Geometry: final body of the model. Coordinates: model frame, mm. A direction names the side the tool comes from. Coordinates: 2 decimals unless noted, no trailing zeros. Order: outer loops, then holes, each group sorted by start corner. A loop starts at its lowest first (then second) coordinate and runs counter-clockwise, first axis right, second up. Notation, with made-up numbers: (73, -4) -> (111, -4) arc R13 ccw to (111, 10) -> close; hole circle Ø5 at (41, 15.25). An arc over 180 degrees is marked (long way). Answer in a Markdown table with one row per item. Add a question column.
1) Set-up query: faces 5 (the face through (-2.41, 1.52, 11.2)), 6 (the face through (-0.066, -3.15, 6.785)), 7 (the face through (0, 2.2, 6.5)). Return all of +Z, -Z, +X, -X, +Y, -Y with unobstructed straight access to the full face (end or side cutting, diameter ignored); none if empty.
2) Section query B-B on z = 2.75. Return the cut outline in (x, y), then the cut area to 3 significant figures.
3) Contact query for flat-ended pins moving along their axis: P1, Ø1.5, axis at x = -3, z = 6.5, coming from the -Y side; P2, Ø1, axis at y = -3.5, z = 2, coming from the -X side; P3, Ø4, axis at x = -3, z = 12.5, coming from the -Y side. Output: stop coordinate, or through.
4) Pull-direction query (X, two-part tool) for faces 1 (the face through (-2.761, -1.518, 6.785)), 2 (the face through (1.95, 0, 3)), 3 (the face through (0, 2.8, 3.2)), 4 (the face through (-3, 3, 6.5)); classes: +X half, -X half, draft (parallel to the pull), parting line (faces both ways), or undercut.
5) Section query A-A on z = 10.25. Return the cut outline in (x, y).
6) Ray query, line 1 (X direction, y = 0, z = 10.5); line 2 (Y direction, x = 0, z = 12); line 3 (Z direction, x = 1.75, y = -4). Return the intervals inside material, ascending. Write a range as from..to.
Autodesk Fusion 360 part; units mm, degrees
sketch "Skizze1" plane through (0, 0, 0) normal (0, 0, 1) x (1, 0, 0)
  circle A0 centre (0, 0) radius 2.8
  circle A1 centre (0, 0) radius 5
  line L0 (1.95, -2.0094) -> (-1.95, -2.0094)
  line L1 (-1.95, -2.0094) -> (-1.95, 2.0094)
  line L2 (-1.95, 2.0094) -> (1.95, 2.0094)
  line L3 (1.95, 2.0094) -> (1.95, -2.0094)
  line L4 (1.95, -2.0094) -> (-1.95, 2.0094) construction
  line L5 (-1.95, -2.0094) -> (1.95, 2.0094) construction
  dimension "d1" = 5.6
  dimension "d2" = 10
  dimension "d3" = 3.9
extrude "Extrusion1" add sketch "Skizze1" along normal blind 6.5 contours A0 L3 | A0 L1 | A1 makes body 1
ref_plane "Arbeitsebene1" through (0, 0, 6.5) normal (0, 0, 1) x (1, 0, 0)
sketch "Skizze2" plane through (0, 0, 6.5) normal (0, 0, 1) x (1, 0, 0)
  line L0 (-3.2893, 0.101) -> (-1.7322, -2.7981)
  line L1 (-1.7322, -2.7981) -> (1.5572, -2.8992)
  line L2 (1.5572, -2.8992) -> (3.2893, -0.101)
  line L3 (3.2893, -0.101) -> (1.7322, 2.7981)
  line L4 (1.7322, 2.7981) -> (-1.5572, 2.8992)
  line L5 (-1.5572, 2.8992) -> (-3.2893, 0.101)
  dimension "d7" = 2.85
extrude "Extrusion2" add sketch "Skizze2" along normal blind 10.5 separate body makes body 2
sketch "Skizze3" plane through (0, 0, 17) normal (0, 0, 1) x (-1, 0, 0)
  line L0 (1.5572, -2.8992) -> (3.2893, -0.101)
  line L1 (3.2893, -0.101) -> (1.7322, 2.7981)
  line L2 (1.7322, 2.7981) -> (-1.5572, 2.8992)
  line L3 (-1.5572, 2.8992) -> (-3.2893, 0.101)
  line L4 (-3.2893, 0.101) -> (-1.7322, -2.7981)
  line L5 (-1.7322, -2.7981) -> (1.5572, -2.8992)
  circle A0 centre (0, 0) radius 2
  dimension "d10" = 4
extrude "Extrusion3" cut sketch "Skizze3" against normal blind 10.5 contours A0 bodies 2
combine "Kombinieren1" operation add target body 1 tool bodies 2
fillet "Abrundung1" radius 1 6 edges at (2.4233, -1.5001, 6.5) (2.5108, 1.3485, 6.5) (0.0875, 2.8487, 6.5) (-0.0875, -2.8487, 6.5) (-2.5108, -1.3485, 6.5) (-2.4233, 1.5001, 6.5) on bodies 1
extrude "Extrusion4" cut 1 faces at (-0.1082, -2.5639, 17) along direction (0, 0, -1) blind 2 on bodies 1 bodies 1
equation "d7 = ( 5.7 / 2 ) * 1 mm"
Result:
| question | item | result |
|---|---|---|
| 1 | face 5 | +Z, -X, +Y |
| 1 | face 6 | +Z, -X, -Y |
| 1 | face 7 | -Z |
| 2 | outline | circle Ø10 at (0, 0); hole (-1.95, -2.01) arc R2.8 ccw to (1.95, -2.01) -> (1.95, 2.01) arc R2.8 ccw to (-1.95, 2.01) -> close |
| 2 | area | 58.6 mm2 |
| 3 | P1 | y = -4.47 |
| 3 | P2 | x = -4 |
| 3 | P3 | y = -2.82 |
| 4 | face 1 | -X half |
| 4 | face 2 | undercut |
| 4 | face 3 | undercut |
| 4 | face 4 | draft |
| 5 | outline | (-3.29, 0.1) -> (-1.73, -2.8) -> (1.56, -2.9) -> (3.29, -0.1) -> (1.73, 2.8) -> (-1.56, 2.9) -> close; hole circle Ø4 at (0, 0) |
| 6 | line 1 | -3.24..-2, 2..3.24 |
| 6 | line 2 | -2.85..-2, 2..2.85 |
| 6 | line 3 | 0..6.5 |
